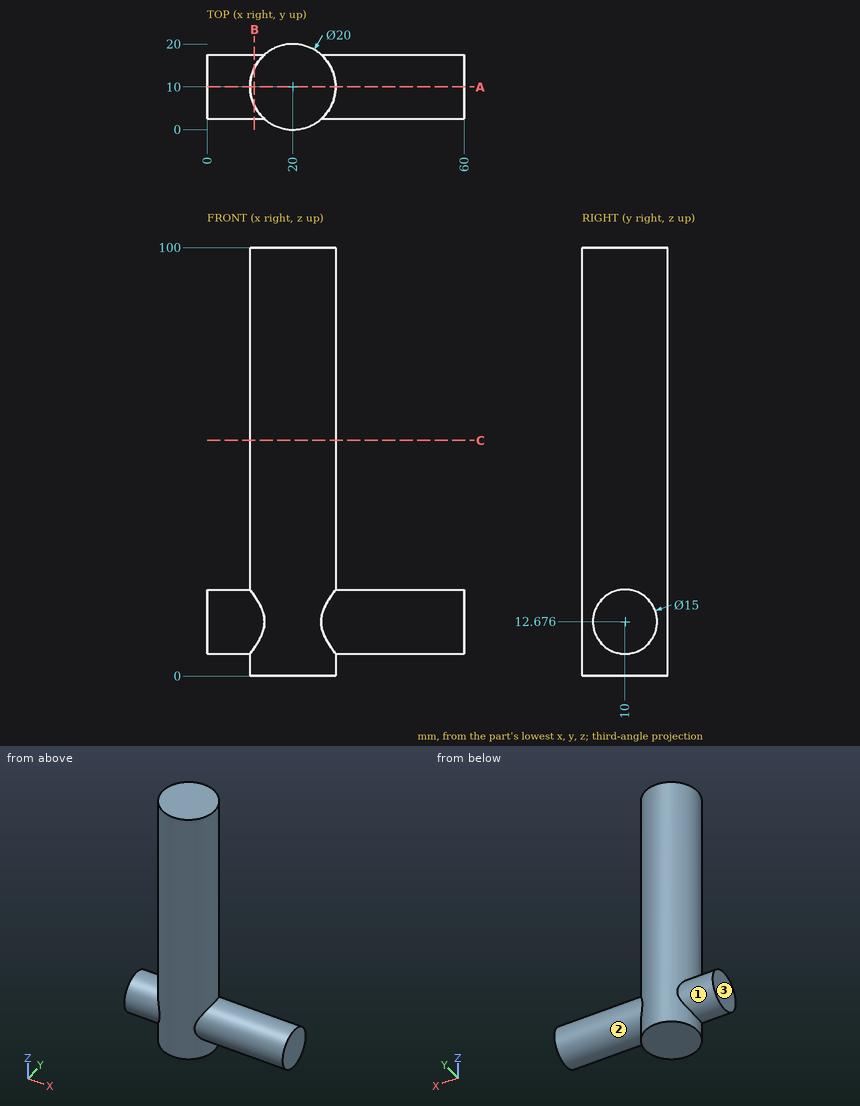
Source: three-view drawing plus pictorial views. Frame: mm from the lowest corner of the part. A direction names the side the tool comes from. Coordinates: 2 decimals unless noted, no trailing zeros. Order: outer loops, then holes, each group sorted by start corner. A loop starts at its lowest first (then second) coordinate and runs counter-clockwise, first axis right, second up. Notation, with made-up numbers: M 0.5,65.5 L 55.5,65.5 A36 ccw 55.5,99.5 Z; hole C -37,-17.75 d4. An arc over 180 degrees is marked long. One line per question, with ' | ' between items. Start each with the question number.
Item 1: Cut plane A-A, the plane y = 10. Return the cut outline in (x, z), then the cut area to 3 significant figures.
Item 2: Cut plane B-B, the plane x = 11. Return the cut outline in (y, z).
Item 3: Ray query, probe 1 along X at (y, z) = (17.5, 15) (1 decimal); probe 2 along Y at (x, z) = (20, 35); probe 3 along X at (y, z) = (15.25, 78.5). Return the intervals inside material, ascending. Write a range as [from, to].
Item 4: Set-up query: the marked faces 1, 2 and 3. Return all of +Z, -Z, +X, -X, +Y, -Y with unobstructed straight access to the full face (end or side cutting, diameter ignored); none if empty.
Item 5: Cut plane C-C, the plane z = 55. Return the cut outline in (x, y), then the cut area to 3 significant figures.
Item 6: Pin query (flat end, axial travel): pin 1 Ø5 at (y, z) = (7, 28.5) entering from +X; pin 2 Ø5 at (y, z) = (17, 43) entering from +X; pin 3 Ø8 at (x, z) = (8, 14.5) entering from +Y. Return the tip coordinate at first contact, or that it passes through.
A:
1) outline: M 0,5.18 L 10,5.18 L 10,0 L 30,0 L 30,5.18 L 60,5.18 L 60,20.18 L 30,20.18 L 30,100 L 10,100 L 10,20.18 L 0,20.18 Z | area: 2,600 mm2
2) outline: M 5.64,0 L 14.36,0 L 14.36,6.57 A7.5 ccw 14.36,18.78 L 14.36,100 L 5.64,100 L 5.64,18.78 A7.5 ccw 5.64,6.57 Z
3) probe 1: x = [13.4, 26.6] | probe 2: y = [0, 20] | probe 3: x = [11.49, 28.51]
4) face 1: -X | face 2: +X | face 3: +Z, -Z, -X, +Y, -Y
5) outline: C 20,10 d20 | area: 314 mm2
6) pin 1: stops at x = 29.99 | pin 2: stops at x = 28.93 | pin 3: stops at y = 17.5
